Here's how the part is built. I have some questions about the finished solid (model axes, mm). Give positions to 0.01 mm unless a question says otherwise; leave off trailing zeros. Order: outer loops, then holes, each group sorted by start corner. A loop starts at its lowest first (then second) coordinate and runs counter-clockwise, first axis right, second up. Notation, with made-up numbers: M 71.5,-22.75 L 92.5,-22.75 A11 cw 92.5,-7.75 Z; hole C 73,86.5 d7. An arc over 180 degrees is marked long. Use CSV: the item, a comma, the result in double quotes. Start each with the question number.
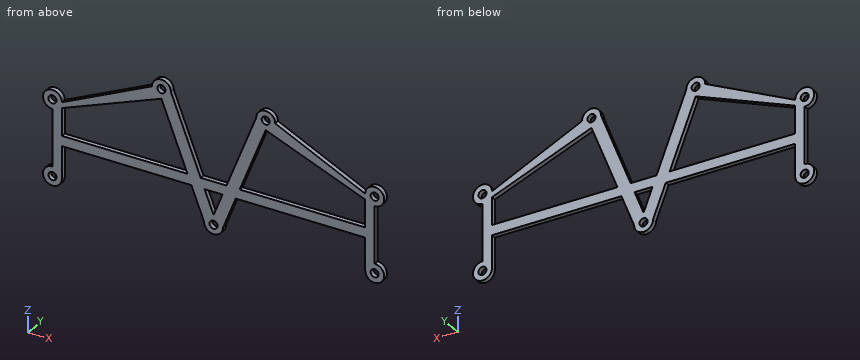
```python
from build123d import *

# Parameters (mm, degrees)
SKETCH1_R           = 1.7
BOSS_EXTRUDE2_DEPTH = 2


with BuildPart() as part:
    # Sketch1 → Boss-Extrude2 (new body)
    with BuildSketch(Plane.XZ.offset(3.574146791)):
        with BuildLine():
            Line((-152.723385358, 44.700516394), (-152.723385358, 20.700516394))
            ThreePointArc((-152.723385358, 20.700516394), (-155.551812483, 13.872089269), (-148.723385358, 16.700516394))
            Line((-148.723385358, 16.700516394), (-148.723385358, 30.384571347))
            Line((-148.723385358, 30.384571347), (-94.078015557, 30.384571347))
            Line((-94.078015557, 30.384571347), (-88.723385358, 16.700516394))
            ThreePointArc((-88.723385358, 16.700516394), (-84.723385358, 12.700516394), (-80.723385358, 16.700516394))
            Line((-80.723385358, 16.700516394), (-75.368755159, 30.384571347))
            Line((-75.368755159, 30.384571347), (-20.723385358, 30.384571347))
            Line((-20.723385358, 30.384571347), (-20.723385358, 16.700516394))
            ThreePointArc((-20.723385358, 16.700516394), (-13.894958233, 13.872089269), (-16.723385358, 20.700516394))
            Line((-16.723385358, 20.700516394), (-16.723385358, 44.700516394))
            ThreePointArc((-16.723385358, 44.700516394), (-13.894958233, 51.528943519), (-20.723385358, 48.700516394))
            Line((-20.723385358, 48.700516394), (-58.723385358, 66.700516394))
            ThreePointArc((-58.723385358, 66.700516394), (-62.723385358, 70.700516394), (-66.723385358, 66.700516394))
            Line((-66.723385358, 66.700516394), (-79.270108033, 34.636669558))
            Line((-79.270108033, 34.636669558), (-90.176662683, 34.636669558))
            Line((-90.176662683, 34.636669558), (-102.723385358, 66.700516394))
            ThreePointArc((-102.723385358, 66.700516394), (-106.723385358, 70.700516394), (-110.723385358, 66.700516394))
            Line((-110.723385358, 66.700516394), (-148.723385358, 48.700516394))
            ThreePointArc((-148.723385358, 48.700516394), (-155.551812483, 51.528943519), (-152.723385358, 44.700516394))
        make_face()
        with Locations(Location((-152.723385358, 48.700516394, 0), (0, 0, 270))):
            Circle(SKETCH1_R, mode=Mode.SUBTRACT)
        with Locations(Location((-106.723385358, 66.700516394, 0), (0, 0, 270))):
            Circle(SKETCH1_R, mode=Mode.SUBTRACT)
        with Locations(Location((-62.723385358, 66.700516394, 0), (0, 0, 270))):
            Circle(SKETCH1_R, mode=Mode.SUBTRACT)
        with Locations(Location((-16.723385358, 48.700516394, 0), (0, 0, 270))):
            Circle(SKETCH1_R, mode=Mode.SUBTRACT)
        with Locations(Location((-152.723385358, 16.700516394, 0), (0, 0, 270))):
            Circle(SKETCH1_R, mode=Mode.SUBTRACT)
        with Locations(Location((-84.723385358, 16.700516394, 0), (0, 0, 270))):
            Circle(SKETCH1_R, mode=Mode.SUBTRACT)
        with Locations(Location((-16.723385358, 16.700516394, 0), (0, 0, 270))):
            Circle(SKETCH1_R, mode=Mode.SUBTRACT)
        Polygon((-148.723385358, 46.265733785), (-148.723385358, 34.636669558), (-95.741880075, 34.636669558), (-106.723385358, 62.700516394), align=None, mode=Mode.SUBTRACT)
        Polygon((-84.723385358, 20.700516394), (-80.933972551, 30.384571347), (-88.512798166, 30.384571347), align=None, mode=Mode.SUBTRACT)
        Polygon((-62.723385358, 62.700516394), (-73.704890642, 34.636669558), (-20.723385358, 34.636669558), (-20.723385358, 46.265733785), align=None, mode=Mode.SUBTRACT)
    extrude(amount=BOSS_EXTRUDE2_DEPTH)


solid = part.part
```
Q1. Imagine slicing it at C-C, the plane x = -70. Please give me the cut outline in (y, z).
Q2. I need wall thicknesses on line 1 (X direction, y = -4, z = 41); line 2 (X direction, y = -4.15, z = 26); line 3 (Z direction, x = -123, y = -5.5). Which ranges of each line are inside material? Lowest first, please. Write a range as [from, to].
Q3. Imagine slicing it at B-B, the plane y = -5.2. Count the separate pieces of the cut face and the enclosed holes in it, then the cut area to 3 significant figures.
Q4. Imagine slicing it at A-A, the plane x = -121. Please give me the cut outline in (y, z), then the cut area to 3 significant figures.
Q5. For P1, Ø1, axis at x = -125, y = -4.5, coming from the +Z side; P2, Ø2, axis at x = -16.72, z = 16.7, coming from the +Y side; P3, Ø1, axis at x = -82.5, y = -4, coming from the +Z side; P4, Ø1, axis at y = -5, z = 34.5, coming from the +X side, each with a flat end and sliding along its axis, tell me the tip position at first contact or that it passes through.
Reply:
1,outline,"M -5.57,30.38 L -3.57,30.38 L -3.57,34.64 L -5.57,34.64 Z; M -5.57,44.1 L -3.57,44.1 L -3.57,58.33 L -5.57,58.33 Z"
2,line 1,"x = [-152.72, -148.72], [-98.23, -92.67], [-76.78, -71.21], [-20.72, -16.72]"
2,line 2,"x = [-152.72, -148.72], [-92.36, -86.8], [-82.65, -77.08], [-20.72, -16.72]"
2,line 3,"z = [30.38, 34.64], [56.33, 60.89]"
3,separate pieces,"1"
3,enclosed holes,"10"
3,area,"1,800 mm^2"
4,outline,"M -5.57,30.38 L -3.57,30.38 L -3.57,34.64 L -5.57,34.64 Z; M -5.57,57.11 L -3.57,57.11 L -3.57,61.83 L -5.57,61.83 Z"
4,area,"17.9 mm^2"
5,P1,"stops at z = 60.17"
5,P2,"passes through"
5,P3,"stops at z = 34.64"
5,P4,"stops at x = -16.72"
